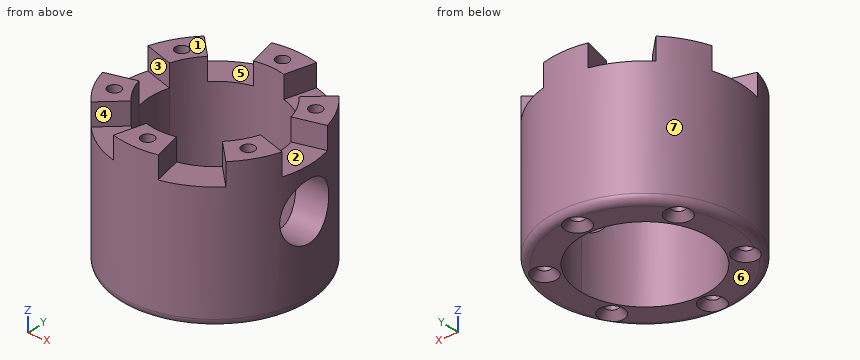
from build123d import *

# Parameters (mm, degrees)
SKETCH1_R                                      = 16.891
BOSS_EXTRUDE1_DEPTH                            = 26.162
SKETCH9_R                                      = 9.525
CUT_EXTRUDE6_DEPTH                             = 36.426854306
SKETCH10_R                                     = 11.43
BOSS_EXTRUDE2_DEPTH                            = 19.05
SKETCH11_R                                     = 9.525
CUT_EXTRUDE7_DEPTH                             = 36.426854306
CUT_EXTRUDE8_DEPTH                             = 3.96875
CSK_FOR_2_FLAT_HEAD_MACHINE_SCREW1_D           = 2.2606
CSK_FOR_2_FLAT_HEAD_MACHINE_SCREW1_CSINK_D     = 4.3688
CSK_FOR_2_FLAT_HEAD_MACHINE_SCREW1_CSINK_ANGLE = 82
CIRPATTERN1_COUNT                              = 6
F_1_2_0_4_DIAMETER_HOLE1_D                     = 10.16
F_1_2_0_4_DIAMETER_HOLE1_DEPTH                 = 12.7
F_1_2_0_4_DIAMETER_HOLE1_TIP                   = 3.052371945
FILLET1_R                                      = 1.27


with BuildPart() as part:
    # Sketch1 → Boss-Extrude1 (new body)
    with BuildSketch(Plane.XY):
        Circle(SKETCH1_R)
    extrude(amount=BOSS_EXTRUDE1_DEPTH)

    # Sketch9 → Cut-Extrude6 (cut, through all)
    with BuildSketch(Plane(origin=(0, 0, 0), x_dir=(-1, 0, 0), z_dir=(0, 0, -1))):
        Circle(SKETCH9_R)
        with BuildLine():
            ThreePointArc((-5.359640753, -7.874), (0, -9.525), (5.359640753, -7.874))
            Line((5.359640753, -7.874), (-5.359640753, -7.874))
        make_face()
        with BuildLine():
            ThreePointArc((-7.874, 5.359640753), (-9.525, 0), (-7.874, -5.359640753))
            Line((-7.874, -5.359640753), (-7.874, 5.359640753))
        make_face()
        with BuildLine():
            Line((-5.359640753, 7.874), (5.359640753, 7.874))
            ThreePointArc((5.359640753, 7.874), (0, 9.525), (-5.359640753, 7.874))
        make_face()
        with BuildLine():
            Line((7.874, 5.359640753), (7.874, -5.359640753))
            ThreePointArc((7.874, -5.359640753), (9.102897204, -2.804084075), (9.525, 0))
            ThreePointArc((9.525, 0), (9.102897204, 2.804084075), (7.874, 5.359640753))
        make_face()
    extrude(amount=-CUT_EXTRUDE6_DEPTH, mode=Mode.SUBTRACT)

    # Sketch10 → Boss-Extrude2 (add)
    # profile 1 of 2: a face of its own
    with BuildSketch(Plane(origin=(0, 0, 0), x_dir=(-1, 0, 0), z_dir=(0, 0, -1))):
        Circle(SKETCH10_R)
        with BuildLine():
            ThreePointArc((-5.359640753, -7.874), (-4.453933477, 8.419507206), (9.525, 0))
            ThreePointArc((9.525, 0), (8.419507206, -4.453933477), (5.359640753, -7.874))
            ThreePointArc((5.359640753, -7.874), (0, -9.525), (-5.359640753, -7.874))
        make_face(mode=Mode.SUBTRACT)
    # profile 2 of 2: a face of its own
    with BuildSketch(Plane(origin=(0, 0, 0), x_dir=(-1, 0, 0), z_dir=(0, 0, -1))):
        Circle(SKETCH10_R)
        with BuildLine():
            ThreePointArc((-5.359640753, -7.874), (-4.453933477, 8.419507206), (9.525, 0))
            ThreePointArc((9.525, 0), (8.419507206, -4.453933477), (5.359640753, -7.874))
            ThreePointArc((5.359640753, -7.874), (0, -9.525), (-5.359640753, -7.874))
        make_face(mode=Mode.SUBTRACT)
    extrude(amount=-BOSS_EXTRUDE2_DEPTH)

    # Sketch11 → Cut-Extrude7 (cut, through all)
    with BuildSketch(Plane.XY.offset(26.162)):
        with BuildLine():
            Line((-9.153468369, -2.634319991), (-10.984162043, -3.161183989))
            ThreePointArc((-10.984162043, -3.161183989), (1.596234295, -11.317991698), (11.43, 0))
            ThreePointArc((11.43, 0), (1.610471515, 11.315974615), (-10.976173491, 3.188810986))
            Line((-10.976173491, 3.188810986), (-9.146811242, 2.657342489))
            ThreePointArc((-9.146811242, 2.657342489), (1.342059596, 9.429978846), (9.525, 0))
            ThreePointArc((9.525, 0), (1.330195246, -9.431659748), (-9.153468369, -2.634319991))
        make_face()
        Circle(SKETCH11_R)
        with BuildLine():
            ThreePointArc((-10.984162043, -3.161183989), (-11.297244321, 0.014212394), (-10.976173491, 3.188810986))
            Line((-10.976173491, 3.188810986), (0, 0))
            Line((0, 0), (-10.984162043, -3.161183989))
        make_face()
        with BuildLine():
            ThreePointArc((-10.976173491, 3.188810986), (-11.429990955, 0.014379395), (-10.984162043, -3.161183989))
            ThreePointArc((-10.984162043, -3.161183989), (-11.297244321, 0.014212394), (-10.976173491, 3.188810986))
        make_face()
    extrude(amount=-CUT_EXTRUDE7_DEPTH, mode=Mode.SUBTRACT)

    # Sketch11<4> → Cut-Extrude8 (cut)
    with BuildSketch(Plane.XY.offset(26.162)):
        with BuildLine():
            ThreePointArc((-10.976173491, 3.188810986), (-11.297244321, 0.014212394), (-10.984162043, -3.161183989))
            Line((-10.984162043, -3.161183989), (0, 0))
            Line((0, 0), (-10.976173491, 3.188810986))
        make_face()
        with BuildLine():
            ThreePointArc((-10.976173491, 3.188810986), (-11.429990955, 0.014379395), (-10.984162043, -3.161183989))
            ThreePointArc((-10.984162043, -3.161183989), (-11.297244321, 0.014212394), (-10.976173491, 3.188810986))
        make_face()
        with BuildLine():
            Line((-16.232150575, -4.67152745), (-10.984162043, -3.161183989))
            ThreePointArc((-10.984162043, -3.161183989), (-11.429990955, 0.014379395), (-10.976173491, 3.188810986))
            Line((-10.976173491, 3.188810986), (-16.220345269, 4.712354013))
            ThreePointArc((-16.220345269, 4.712354013), (-16.925737574, 0.021293268), (-16.232150575, -4.67152745))
        make_face()
        with BuildLine():
            Line((0, 0), (-10.984162043, -3.161183989))
            ThreePointArc((-10.984162043, -3.161183989), (1.596234295, -11.317991698), (11.43, 0))
            ThreePointArc((11.43, 0), (1.610471515, 11.315974615), (-10.976173491, 3.188810986))
            Line((-10.976173491, 3.188810986), (0, 0))
        make_face()
    cut_extrude8 = extrude(amount=-CUT_EXTRUDE8_DEPTH, mode=Mode.SUBTRACT)

    # CSK for #2 Flat Head Machine Screw1 (through all)
    with Locations(Plane(origin=(0, 0, 0), x_dir=(-1, 0, 0), z_dir=(0, 0, -1))):
        with Locations((12.089577909, 7.000214709)):
            csk_for_2_flat_head_machine_screw1 = CounterSinkHole(CSK_FOR_2_FLAT_HEAD_MACHINE_SCREW1_D / 2, CSK_FOR_2_FLAT_HEAD_MACHINE_SCREW1_CSINK_D / 2, counter_sink_angle=CSK_FOR_2_FLAT_HEAD_MACHINE_SCREW1_CSINK_ANGLE)

    # CirPattern1: Cut-Extrude8, CSK for #2 Flat Head Machine Screw1 ×6 about axis
    cirpattern1_axis = Axis((0, 0, 0), (0, 0, 1))
    add([cut_extrude8.rotate(cirpattern1_axis, i * 360 / CIRPATTERN1_COUNT) for i in range(1, CIRPATTERN1_COUNT)], mode=Mode.SUBTRACT)
    add([csk_for_2_flat_head_machine_screw1.rotate(cirpattern1_axis, i * 360 / CIRPATTERN1_COUNT) for i in range(1, CIRPATTERN1_COUNT)], mode=Mode.SUBTRACT)

    # 1/2 (0.4) Diameter Hole1
    with Locations(Plane(origin=(16.890986634, -0.02124955, 14.908061188), x_dir=(0.001258039772, 0.999999208668, 0), z_dir=(0.999999208668, -0.001258039772, 0))):
        with Locations((0, 0)):
            Hole(F_1_2_0_4_DIAMETER_HOLE1_D / 2, depth=F_1_2_0_4_DIAMETER_HOLE1_DEPTH)
            with Locations((0, 0, -(F_1_2_0_4_DIAMETER_HOLE1_DEPTH + F_1_2_0_4_DIAMETER_HOLE1_TIP / 2))):  # 118° drill point
                Cone(0, F_1_2_0_4_DIAMETER_HOLE1_D / 2, F_1_2_0_4_DIAMETER_HOLE1_TIP, mode=Mode.SUBTRACT)

    # Fillet1
    # the kernel refuses this fillet: 1.27 mm, written as the material it takes off along each edge
    with BuildSketch(Plane(origin=(0, 0, 0), x_dir=(1, 0, 0), z_dir=(0, -1, 0))) as fillet1_piece_1:
        with BuildLine():
            CenterArc((16.891 - FILLET1_R, FILLET1_R), FILLET1_R, 270, 90)
            Line((16.891 - FILLET1_R, 0), (16.891, 0))
            Line((16.891, 0), (16.891, FILLET1_R))
        make_face()
    revolve(axis=Axis((0, 0, 0), (0, 0, 1)), mode=Mode.SUBTRACT)


solid = part.part
Input: part model. Units: mm. Frame: model coordinates. Face numbers are marked on the shaded views. A direction names the side the tool comes from. Give positions to 0.01 mm unless a question says otherwise; leave off trailing zeros. Order: outer loops, then holes, each group sorted by start corner. A loop starts at its lowest first (then second) coordinate and runs counter-clockwise, first axis right, second up. Notation, with made-up numbers: (50, 16) - (70, 16) arc R17 cw to (70, 39) - close; hole circle Ø4 at (-14.75, 23.5). An arc over 180 degrees is marked (long way). Answer as a JSON object with one key per item and string values. Group by question number.
Q1. Cut plane D-D, the plane z = 17. Output: boundary loops of the cut face in (x, y), then the cut area to 3 significant figures.
Q2. Set-up query: the marked faces 1, 2 and 3. Return all of +Z, -Z, +X, -X, +Y, -Y with unobstructed straight access to the full face (end or side cutting, diameter ignored); none if empty.
Q3. Line query: probe 1 along Y at (x, z) = (0, 20.25); probe 2 along Y at (x, z) = (-8.5, 20.75); probe 3 along X at (y, z) = (7.5, 16.5). Output: solid intervals per line, ascending.
Q4. Cut plane A-A, the plane z = 13.5. Output: boundary loops of the cut face in (x, y).
Q5. Cut plane C-C, the plane x = 0. Count the separate pieces of the cut face and the enclosed holes in it, then the cut area to 3 significant figures.
Q6. First-contact query: pin 1 Ø2 at (y, z) = (-0.5, 16.5) entering from +X; pin 2 Ø4 at (x, y) = (-9.5, -11) entering from +Z; pin 3 Ø10 at (x, z) = (6, 11) entering from -Y; pin 4 Ø8 at (x, z) = (-5.5, 3.5) entering from -Y. Flat tips, straight axial feed; report the tip coordinate or a pass-through.
Q7. Mould query, pull axis X, two halves, no side actions, for the marked faces 4, 5, 6 and 7. Classes: pulls with the +X half, pulls with the -X half, needs draft (parallel to the pull), parting line crosses it, or undercut.
Q8. Cut plane B-B, the plane z = 6.75. Output: boundary loops of the cut face in (x, y).
Results:
{
 "1": {"outline": "(10.44, -4.64) arc R11.43 cw (long way) to (10.46, 4.62) - (16.25, 4.61) arc R16.89 ccw (long way) to (16.24, -4.65) - close; hole circle Ø2.26 at (-12.11, -6.97); hole circle Ø2.26 at (-12.09, 7); hole circle Ø2.26 at (-0.02, -13.97); hole circle Ø2.26 at (0.02, 13.97); hole circle Ø2.26 at (12.09, -7); hole circle Ø2.26 at (12.11, 6.97)", "area": "410 mm^2"},
 "2": {"face 1": "+Z, +X, -X, +Y, -Y", "face 2": "+Z, +X", "face 3": "+Z, -X"},
 "3": {"probe 1": "-16.89 to -15.1, -12.84 to -11.43, 11.43 to 12.84, 15.1 to 16.89", "probe 2": "-14.6 to -7.64, 7.64 to 14.6", "probe 3": "-15.13 to -13.1, -11.08 to -8.63, 8.63 to 11.11, 13.11 to 15.13"},
 "4": {"outline": "(10.33, -4.89) arc R11.43 cw (long way) to (10.34, 4.87) - (16.18, 4.86) arc R16.89 ccw (long way) to (16.16, -4.9) - close; hole circle Ø2.26 at (-12.11, -6.97); hole circle Ø2.26 at (-12.09, 7); hole circle Ø2.26 at (-0.02, -13.97); hole circle Ø2.26 at (0.02, 13.97); hole circle Ø2.26 at (12.09, -7); hole circle Ø2.26 at (12.11, 6.97)"},
 "5": {"separate pieces": "4", "enclosed holes": "0", "area": "164 mm^2"},
 "6": {"pin 1": "x = -11.33", "pin 2": "z = 26.16", "pin 3": "y = -16.86", "pin 4": "y = -16.82"},
 "7": {"face 4": "undercut", "face 5": "undercut", "face 6": "needs draft", "face 7": "parting line crosses it"},
 "8": {"outline": "circle Ø33.78 at (0, 0); hole circle Ø2.26 at (-12.11, -6.97); hole circle Ø2.26 at (-12.09, 7); hole circle Ø22.86 at (0, 0); hole circle Ø2.26 at (-0.02, -13.97); hole circle Ø2.26 at (0.02, 13.97); hole circle Ø2.26 at (12.09, -7); hole circle Ø2.26 at (12.11, 6.97)"}
}
